Source: CAD feature listing. Evaluate the final solid. Frame: model axes, mm. A direction names the side the tool comes from. Round coordinates to 2 decimals unless told otherwise and drop trailing zeros. Write each loop counter-clockwise with the first axis right and the second up, starting at its lowest first coordinate (ties: lowest second). Pieces come first, ordered by that corner, then holes. Notation, with made-up numbers: M 23.5,1 L 70.5,1 A28 ccw 70.5,32 Z; hole C 56.5,69 d1. An arc over 180 degrees is marked long. Answer in a Markdown table with one row per item.
from build123d import *
from build123d.topology import SkipClean

# Parameters (mm, degrees)
SKETCH1_R           = 2.5
BOSS_EXTRUDE1_DEPTH = 2.3
BOSS_EXTRUDE2_START = 2.7
SKETCH2_R           = 2.5
BOSS_EXTRUDE2_DEPTH = 2.7
SKETCH3_R           = 2.5
CUT_EXTRUDE1_DEPTH  = 10
BOSS_EXTRUDE3_START = -5
SKETCH4_R           = 2.5
BOSS_EXTRUDE3_DEPTH = 5
SKETCH4_3_R         = 2.5
CUT_EXTRUDE2_DEPTH  = 5


with BuildPart() as part:
    # Sketch1 → Boss-Extrude1 (new body)
    with BuildSketch(Plane(origin=(0, 0, 0), x_dir=(0, 0, -1), z_dir=(1, 0, 0))):
        with BuildLine():
            Line((-16.5, -7.5), (20.481500629, -7.48452785))
            ThreePointArc((20.481500629, -7.48452785), (27.496130965, 0.240874575), (20, 7.5))
            Line((20, 7.5), (-16.5, 7.5))
            ThreePointArc((-16.5, 7.5), (-24, 0), (-16.5, -7.5))
        make_face()
        with BuildLine():
            Line((4.012796555, 4.594285996), (10.45821766, 3.581381658))
            Line((10.45821766, 3.581381658), (10.45821766, 0))
            Line((10.45821766, 0), (10.45821766, -3.581381658))
            Line((10.45821766, -3.581381658), (4.012796555, -4.594285996))
            ThreePointArc((4.012796555, -4.594285996), (0, -6.1), (-4.012796555, -4.594285996))
            Line((-4.012796555, -4.594285996), (-9.954017871, -3.660617157))
            Line((-9.954017871, -3.660617157), (-16.903638766, -2.568477321))
            ThreePointArc((-16.903638766, -2.568477321), (-19.1, 0), (-16.903638766, 2.568477321))
            Line((-16.903638766, 2.568477321), (-4.012796555, 4.594285996))
            ThreePointArc((-4.012796555, 4.594285996), (0, 6.1), (4.012796555, 4.594285996))
        make_face(mode=Mode.SUBTRACT)
        with Locations((20, 0)):
            Circle(SKETCH1_R, mode=Mode.SUBTRACT)
    extrude(amount=BOSS_EXTRUDE1_DEPTH)

    # Sketch2 → Boss-Extrude2 (add)
    with SkipClean():  # the faces are left unmerged after this step: merging them gives an invalid solid
        with BuildSketch(Plane.ZY.offset(BOSS_EXTRUDE2_START)):
            with BuildLine():
                Line((16.5, 7.5), (-20, 7.5))
                ThreePointArc((-20, 7.5), (-27.496130965, 0.240874575), (-20.481500629, -7.48452785))
                Line((-20.481500629, -7.48452785), (16.5, -7.5))
                ThreePointArc((16.5, -7.5), (24, 0), (16.5, 7.5))
            make_face()
            with Locations((-20, 0)):
                Circle(SKETCH2_R, mode=Mode.SUBTRACT)
        extrude(amount=-BOSS_EXTRUDE2_DEPTH)

    # Sketch3 → Cut-Extrude1 (cut)
    with SkipClean():  # the faces are left unmerged after this step: merging them gives an invalid solid
        with BuildSketch(Plane(origin=(0, 0, 0), x_dir=(0, 0, -1), z_dir=(1, 0, 0))):
            Circle(SKETCH3_R)
        extrude(amount=-CUT_EXTRUDE1_DEPTH, mode=Mode.SUBTRACT)

    # Sketch4 → Boss-Extrude3 (add)
    with BuildSketch(Plane(origin=(2.3, 0, 0), x_dir=(0, 0, -1), z_dir=(1, 0, 0)).offset(BOSS_EXTRUDE3_START)):
        with BuildLine():
            ThreePointArc((25.481500629, -7.48452785), (32.496130965, 0.240874575), (25, 7.5))
            Line((25, 7.5), (20, 7.5))
            ThreePointArc((20, 7.5), (27.496130965, 0.240874575), (20.481500629, -7.48452785))
            Line((20.481500629, -7.48452785), (25.481500629, -7.48452785))
        make_face()
        with Locations((20, 0)):
            Circle(SKETCH4_R)
    extrude(amount=BOSS_EXTRUDE3_DEPTH)

    # Sketch4_3 → Cut-Extrude2 (cut)
    with BuildSketch(Plane(origin=(2.3, 0, 0), x_dir=(0, 0, -1), z_dir=(1, 0, 0))):
        with Locations((25, 0)):
            Circle(SKETCH4_3_R)
    extrude(amount=-CUT_EXTRUDE2_DEPTH, mode=Mode.SUBTRACT)


solid = part.part
Q1. Contact query for flat-ended pins moving along their axis: pin 1 Ø0.7 at (x, y) = (1, 1.5) entering from +Z; pin 2 Ø1.5 at (x, y) = (-1.5, 5.5) entering from +Z; pin 3 Ø6 at (y, z) = (0, 0) entering from -X. Output: stop coordinate, or through.
Solutions:
| item | result |
|---|---|
| pin 1 | stops at z = 23.91 |
| pin 2 | stops at z = 22.3 |
| pin 3 | stops at x = -2.7 |
Q2. Section C-C (z = 0). Return loops of the section in (x, y), and give its area (3 significant figures).
Solutions:
| item | result |
|---|---|
| outline | M -2.7,-7.49 L 2.3,-7.49 L 2.3,-6.1 L 0,-6.1 L 0,-2.5 L -2.7,-2.5 Z; M -2.7,2.5 L 0,2.5 L 0,6.1 L 2.3,6.1 L 2.3,7.5 L -2.7,7.5 Z |
| area | 33.4 mm2 |
Q3. Section D-D (z = 15.5). Return loops of the section in (x, y).
Solutions:
| item | result |
|---|---|
| outline | M -2.7,-7.5 L 2.3,-7.5 L 2.3,-2.79 L 0,-2.79 L 0,2.79 L 2.3,2.79 L 2.3,7.5 L -2.7,7.5 Z |
Q4. Pull-direction query (Z, two-part tool) for faces 1 (the cylindrical face through (-0.2, 0.1, -32.5)), 2 (the flat face through (0, 0, 4)), 3 (the cylindrical face through (0, 0, 24)); classes: pulls with the +Z half, pulls with the -Z half, needs draft (parallel to the pull), parting line crosses it, or undercut.
Solutions:
| item | result |
|---|---|
| face 1 | pulls with the -Z half |
| face 2 | undercut |
| face 3 | pulls with the +Z half |
Q5. Material intervals for probe 1 along Y at (x, z) = (-2.05, 0); probe 2 along Z at (x, y) = (1.3, 0.5); probe 3 along Y at (x, z) = (-1.95, 5), sorted ascending.
Solutions:
| item | result |
|---|---|
| probe 1 | y = -7.49 to -2.5, 2.5 to 7.5 |
| probe 2 | z = -32.48 to -27.45, -22.55 to -10.46, 19.05 to 23.98 |
| probe 3 | y = -7.5 to 7.5 |
Q6. Section B-B (y = 0). Return loops of the section in (x, z).
Solutions:
| item | result |
|---|---|
| outline | M -2.7,-32.5 L 2.3,-32.5 L 2.3,-27.5 L -2.7,-27.5 Z; M -2.7,-22.5 L 2.3,-22.5 L 2.3,-10.46 L 0,-10.46 L 0,-2.5 L -2.7,-2.5 Z; M -2.7,2.5 L 0,2.5 L 0,19.1 L 2.3,19.1 L 2.3,24 L -2.7,24 Z |
Q7. Section A-A (x = 0.85). Return loops of the section in (y, z).
Solutions:
| item | result |
|---|---|
| outline | M -7.5,16.5 L -7.48,-20.48 L -7.48,-25.48 A7.5 ccw 7.5,-25 L 7.5,16.5 A7.5 ccw Z; hole M -4.59,-4.01 L -3.58,-10.46 L 3.58,-10.46 L 4.59,-4.01 A6.1 ccw 4.59,4.01 L 2.57,16.9 A2.6 ccw -2.57,16.9 L -4.59,4.01 A6.1 ccw Z; hole C 0,-25 d5 |
Q8. Access query for faces 4 (the flat face through (1, 0, -10.458)), 5 (the flat face through (2.3, -5, -4)). Directions: +Z, -Z, +X, -X, +Y, -Y. A direction counts if a zero-diameter tool reaches every point of the face in a straight line with its end or side. Return the directions, or none.
Solutions:
| item | result |
|---|---|
| face 4 | +X |
| face 5 | +Z, -Z, +X, +Y, -Y |
